Here's how the part is built. I have some questions about the finished solid (model axes, mm). A direction names the side the tool comes from. Coordinates: 2 decimals unless noted, no trailing zeros. Write each loop counter-clockwise with the first axis right and the second up, starting at its lowest first coordinate (ties: lowest second). Pieces come first, ordered by that corner, then holes. Notation, with made-up numbers: (-7, -33) -> (36, -33) arc R17 ccw to (36, -1) -> close; hole circle Ø5 at (75.25, 35). An arc over 180 degrees is marked (long way). Put each result on its own line as item: value.
Autodesk Inventor part; units mm, degrees
ref_plane "YZ Plane" through (0, 0, 0) normal (1, 0, 0) x (0, 1, 0)
ref_plane "XZ Plane" through (0, 0, 0) normal (0, 1, 0) x (-1, 0, 0)
ref_plane "XY Plane" through (0, 0, 0) normal (0, 0, 1) x (1, 0, 0)
sketch "Sketch1" plane through (0, 0, 0) normal (0, 0, 1) x (1, 0, 0)
  line L0 (0, 0) -> (50, 0)
  line L1 (50, 0) -> (50, 40)
  line L2 (50, 40) -> (0, 40)
  line L3 (0, 40) -> (0, 0)
  dimension "d0" = 50
  dimension "d1" = 40
extrude "Extrusion1" add sketch "Sketch1" along normal blind 70
sketch "Sketch2" plane through (50, 0, 0) normal (1, 0, 0) x (0, 0, -1)
  line L0 (0, 0) -> (0, 40)
  line L1 (0, 40) -> (-70, 40)
  line L2 (-70, 0) -> (-70, 40)
  line L3 (0, 0) -> (-70, 0)
  line L4 (-70, 0) -> (-5, 0)
  line L5 (-5, 0) -> (-5, 22)
  line L6 (-5, 22) -> (-70, 22)
  line L7 (-70, 22) -> (-70, 0)
  point P0 (0, 0)
  dimension "d5" = 5
  dimension "d6" = 18
extrude "Extrusion2" cut sketch "Sketch2" against normal up to next contours L3 L2 L6 L5
sketch "Sketch3" plane through (0, 0, 70) normal (0, 0, 1) x (1, 0, 0)
  line L0 (0, 22) -> (50, 22)
  line L1 (50, 22) -> (50, 40)
  line L2 (50, 40) -> (0, 40)
  line L3 (0, 40) -> (0, 22)
  circle A0 centre (10, 31) radius 4.25
  circle A1 centre (40, 31) radius 4.25
  point P0 (0, 0)
  dimension "d9" = 8.5
  dimension "d10" = 8.5
  dimension "d11" = 30
  dimension "d12" = 50
  dimension "d13" = 10
  dimension "d14" = 18
  dimension "d15" = 9
  dimension "d16" = 9
extrude "Extrusion3" cut sketch "Sketch3" against normal up to next contours A0 | A1
fillet "Fillet1" radius 4 1 edges at (25, 22, 5)
sketch "Sketch4" plane through (0, 0, 0) normal (0, 0, -1) x (-1, 0, 0)
  circle A0 centre (-10, 31) radius 4.25
  circle A1 centre (-40, 31) radius 4.25
  line L0 (0, 0) -> (-50, 0)
  line L1 (0, 40) -> (0, 0)
  line L2 (-50, 40) -> (0, 40)
  line L3 (-50, 0) -> (-50, 40)
  circle A2 centre (-42.175, 7) radius 2.5
  circle A3 centre (-7.825, 7) radius 2.5
  dimension "d20" = 50
  dimension "d21" = 5
  dimension "d22" = 5
  dimension "d23" = 34.35
  dimension "d24" = 7.825
  dimension "d25" = 7
  dimension "d26" = 7
extrude "Extrusion4" cut sketch "Sketch4" against normal up to next contours A2 | A3
fillet "Fillet2" radius 6 4 edges at (35.75, 31, 0) (5.75, 31, 0) (35.75, 31, 70) (5.75, 31, 70)
equation "\"d9\" = d10"
equation "\"d13\" = -0.5 * d11 + 0.5 * d12"
equation "\"d15\" = 0.5 * d14"
equation "\"d16\" = d15"
equation "\"d24\" = -0.5 * d23 + 0.5 * d20"
equation "\"d26\" = d25"
properties part number "tubing_alignment_arm[3]"
Item 1: Imagine slicing it at C-C on x = 28.5. Write out the boundary of the cut face in (y, z).
Output:
outline: (0, 0) -> (40, 0) -> (40, 70) -> (22, 70) -> (22, 9) arc R4 cw to (18, 5) -> (0, 5) -> close
Item 2: Imagine slicing it at D-D on y = 31. Write out the boundary of the cut face in (x, z), then the cut area to 3 significant figures.
Output:
outline: (0, 0.01) arc R6 ccw to (5.75, 6) -> (5.75, 64) arc R6 ccw to (0, 69.99) -> close; (14.25, 6) arc R6 ccw to (20.25, 0) -> (29.75, 0) arc R6 ccw to (35.75, 6) -> (35.75, 64) arc R6 ccw to (29.75, 70) -> (20.25, 70) arc R6 ccw to (14.25, 64) -> close; (44.25, 6) arc R6 ccw to (50, 0.01) -> (50, 69.99) arc R6 ccw to (44.25, 64) -> close
area: 2,250 mm²
Item 3: Please list where these lines run through material, in increasing order: line 1 along Y through (x, z) = (10, 28); line 2 along X through (y, z) = (29, 15.5); line 3 along Y through (x, z) = (18, 42). Write a range as from..to.
Output:
line 1: y = 22..26.75, 35.25..40
line 2: x = 0..6.25, 13.75..36.25, 43.75..50
line 3: y = 22..40
Item 4: Imagine slicing it at B-B on z = 58. Write out the boundary of the cut face in (x, y), then the cut area to 3 significant figures.
Output:
outline: (0, 22) -> (50, 22) -> (50, 40) -> (0, 40) -> close; hole circle Ø8.5 at (10, 31); hole circle Ø8.5 at (40, 31)
area: 787 mm²
Item 5: Imagine slicing it at A-A on y = 7. Write out the boundary of the cut face in (x, z) (3 decimals).
Output:
outline: (0, 0) -> (5.325, 0) -> (5.325, 5) -> (0, 5) -> close; (10.325, 0) -> (39.675, 0) -> (39.675, 5) -> (10.325, 5) -> close; (44.675, 0) -> (50, 0) -> (50, 5) -> (44.675, 5) -> close
Item 6: Which directions (+Z, -Z, +X, -X, +Y, -Y) give clear straight access to the entire face, cutting with the end or side of a thin tool? Please do faces 1 (the flat face through (25, 9, 5)), 2 (the flat face through (25, 40, 35)).
Output:
face 1: +Z, +X, -X, -Y
face 2: +Z, -Z, +X, -X, +Y
Item 7: If we mould it in two halves opening along X, with no side actions, what happens to faces 3 (the cylindrical face through (5.516, 6.042, 2.465)), 4 (the flat face through (25, 22, 39)), 5 (the cylindrical face through (6.63, 28.41, 35.41)), 6 (the flat face through (50, 29, 35))? For each: released by +X, released by -X, zero draft, split by the parting line, or undercut.
Output:
face 3: undercut
face 4: zero draft
face 5: undercut
face 6: released by +X
Item 8: For P1, Ø13.5, axis at x = 40, y = 31, coming from the +Z side; P2, Ø7.5, axis at x = 10, y = 31, coming from the +Z side; P3, Ø9, axis at x = 25.5, y = 9.5, coming from the +Z side, each with a flat end and sliding along its axis, tell me the tip position at first contact or that it passes through.
Output:
P1: stops at z = 68.87
P2: passes through
P3: stops at z = 5
